Source: CAD feature listing. Evaluate the final solid. Frame: model axes, mm. A direction names the side the tool comes from. Give positions to 0.01 mm unless a question says otherwise; leave off trailing zeros. Loops run counter-clockwise (first coordinate to the right, second up) from the corner with the lowest first, then second, coordinate; pieces in that order, holes last. Notation, with made-up numbers: (-38.5, -18.5) -> (0.5, -18.5) arc R22 ccw to (0.5, -6.5) -> close; hole circle Ø7 at (72.25, 64.25). An arc over 180 degrees is marked (long way). Return JSON: item names as keys, results as strings. Group by question number.
(1) Cut plane D-D on y = -8. Return loops of the section in (x, z), then the cut area to 3 significant figures.
(2) Access query for faces 1 (the face through (0, -19, 24)), 2 (the face through (0, -21, 28)), 3 (the face through (0, 0, 54)). Directions: +Z, -Z, +X, -X, +Y, -Y. A direction counts if a zero-diameter tool reaches every point of the face in a straight line with its end or side. Return the directions, or none.
(3) Draft query along Z for faces 4 (the face through (0, -12.6, 11.5)), 5 (the face through (0, -20, 12)), 6 (the face through (0, -15, 57)). Return one class per face: released by +Z, released by -Z, zero draft, split by the parting line, or undercut.
(4) Cut plane B-B on x = 1.85. Give the number of separate pieces and of enclosed holes in the cut face, then the cut area to 3 significant figures.
(5) Cut plane A-A on y = -15. Return loops of the section in (x, z).
(6) Ray query, line 1 (Y direction, x = -1.1, z = 22.5); line 2 (Y direction, x = -0.05, z = 17); line 3 (Z direction, x = -2.1, y = -9). Return the intervals inside material, ascending. Write a range as from..to.
(7) Pin query (flat end, axial travel): pin 1 (1.5 mm diameter, centred on x = 1.5, z = 50.5, fed in from +Y); pin 2 (2 mm diameter, centred on x = 0, z = 33, fed in from +Y); pin 3 (3 mm diameter, centred on x = 1, z = 29.5, fed in from +Y). Return the tip coordinate at first contact, or that it passes through.
(8) Cut plane C-C on z = 23. Return loops of the section in (x, y), then the cut area to 3 significant figures.
Autodesk Inventor part; units mm, degrees
ref_plane "YZ Plane" through (0, 0, 0) normal (1, 0, 0) x (0, 1, 0)
ref_plane "XZ Plane" through (0, 0, 0) normal (0, 1, 0) x (-1, 0, 0)
ref_plane "XY Plane" through (0, 0, 0) normal (0, 0, 1) x (1, 0, 0)
sketch "Skizze1" plane through (0, 0, 0) normal (1, 0, 0) x (0, 1, 0)
  circle A0 centre (-22.8, 48.7) radius 11 construction
  line L0 (-97.7565, 0) -> (58.6427, 0)
  circle A1 centre (14.8, 21.5) radius 21.5 construction
  line L1 (0, 10) -> (0, 33.674) construction
  line L2 (-6.7, 0) -> (-6.7, 21.5) construction
  circle A2 centre (-4.5, 42.5) radius 5 construction
  line L3 (-56.6136, 29) -> (0, 29) construction
  line L4 (-75.4137, 30) -> (0, 30) construction
  line L5 (-21, 43.3983) -> (-29, 49)
  line L6 (-29, 49) -> (-29, 57)
  circle A3 centre (-4.5, 42.5) radius 5.5
  circle A4 centre (-22.8, 48.7) radius 0.5
  circle A5 centre (-3, 23) radius 0.8
  line L7 (14.8, 21.5) -> (-6.7, 21.5) construction
  line L8 (-29, 57) -> (0, 57)
  line L9 (14.8, 21.5) -> (14.8, 20.5) construction
  line L10 (14.8, 20.5) -> (-4.5, 42.5) construction
  circle A6 centre (-22.8, 48.7) radius 4.95 construction
  circle A7 centre (-12.2958, 49.6823) radius 5.6 construction
  circle A8 centre (-12.2958, 49.6823) radius 6.3 construction
  circle A9 centre (-12.2958, 49.6823) radius 1.525
  line L11 (0, 50.374) -> (0, 57)
  line L12 (-21, 43.3983) -> (-21, 10)
  line L13 (-21, 10) -> (0, 10)
  arc A10 (1.9876, 42.0983) -> (1.2121, 45.6019) centre (-4.5, 42.5) ccw
  line L14 (1.9876, 42.0983) -> (0, 10)
  arc A11 (0, 50.374) -> (1.2121, 45.6019) centre (10, 50.374) ccw
  line L15 (-12.5, 18) -> (-12.5, 31) construction
  line L16 (-19, 18) -> (-19, 31)
  line L17 (-6, 31) -> (-6, 18)
  arc A12 (-19, 18) -> (-6, 18) centre (-12.5, 18) ccw
  arc A13 (-6, 31) -> (-19, 31) centre (-12.5, 31) ccw
  point P0 (0, 0)
  point P1 (-12.5, 24.5)
  dimension "d4" = 43
  dimension "d0" = 22
  dimension "d6" = 6.7
  dimension "d8" = 10
  dimension "d9" = 29
  dimension "d11" = 30
  dimension "d19" = 29
  dimension "d20" = 11
  dimension "d33" = 1
  dimension "d34" = 48.7
  dimension "d36" = 1.6
  dimension "d37" = 3
  dimension "d54" = 57
  dimension "d58" = 1
  dimension "d65" = 9.9
  dimension "d66" = 11.2
  dimension "d67" = 0.7
  dimension "d68" = 3.05
  dimension "d73" = 22.8
  dimension "d100" = 10.5042
  dimension "d101" = 0.9823
  dimension "d102" = 0
  dimension "d103" = 8.3
  dimension "d104" = 21
  dimension "d107" = 10
  dimension "d110" = 8
  dimension "d111" = 55
  dimension "d112" = 13
  dimension "d113" = 10
  dimension "d114" = 42.5
  dimension "d115" = 34
  dimension "d116" = 21
  dimension "d131" = 13
  dimension "d132" = 13
  dimension "d133" = 12.5
  dimension "d134" = 18
  dimension "d135" = 4.5
  dimension "d136" = 10.55
extrude "Extrusion1" add sketch "Skizze1" along normal mid plane 5 contours L5 L6 L8 L11 A11 A10 L14 L13 L12 | A4
sketch "Skizze2" plane through (-2.5, -29, 57) normal (0, 0, 1) x (1, 0, 0)
  line L0 (0, 0) -> (5, 0)
  line L1 (5, 5) -> (5, 0)
  line L2 (0, 0) -> (0, 5)
  line L3 (2.5, 29) -> (2.5, 0) construction
  line L4 (0, 0) -> (5, 0) construction
  line L5 (0, 5) -> (5, 5)
  line L6 (0, 29) -> (5, 29)
  line L7 (0, 29) -> (5, 29)
  point P0 (2.5, 26)
  point P1 (2.5, 3)
  dimension "d25" = 23
  dimension "d74" = 3
hole "Bohrung1" at (0, -3, 57) at (0, -26, 57) direction (0, 0, -1) diameter 2.459 depth 7 tip angle 118
sketch "Skizze3" plane through (-2.5, 0, 0) normal (-1, 0, 0) x (0, 0, 1)
  circle A0 centre (23, -3) radius 0.8
  line L0 (29, -4) -> (17, -4) construction
  circle A1 centre (23, -3) radius 0.8 construction
  line L1 (23, -4) -> (23, -3) construction
  point P0 (0, 0)
  point P1 (55, -8)
  dimension "d38" = 12
  dimension "d39" = 1
  dimension "d40" = 32
  dimension "d41" = 5
hole "Bohrung2" at (-2.5, -4, 17) at (-2.5, -4, 29) at (-2.5, -8, 55) direction (1, 0, 0) diameter 1.567 end through all
fillet "Rundung3" radius 5 4 edges at (0, 0, 10) (0, -21, 10) (0, -21, 43.3983) (0, -29, 49)
properties part number "Dribbler Seite v2" material "Aluminium 6061"
Answers:
{
 "1": {"outline": "(-2.5, 10) -> (2.5, 10) -> (2.5, 13.31) -> (-2.5, 13.31) -> close; (-2.5, 35.69) -> (2.5, 35.69) -> (2.5, 38.26) -> (-2.5, 38.26) -> close; (-2.5, 46.74) -> (2.5, 46.74) -> (2.5, 54.22) -> (-2.5, 54.22) -> close; (-2.5, 55.78) -> (2.5, 55.78) -> (2.5, 57) -> (-2.5, 57) -> close", "area": "72.8 mm²"},
 "2": {"face 1": "+X, -X", "face 2": "-Z, +X, -X, -Y", "face 3": "+Z, +X, -X, +Y"},
 "3": {"face 4": "undercut", "face 5": "released by -Z", "face 6": "released by +Z"},
 "4": {"separate pieces": "1", "enclosed holes": "7", "area": "692 mm²"},
 "5": {"outline": "(-2.5, 10) -> (2.5, 10) -> (2.5, 12) -> (-2.5, 12) -> close; (-2.5, 37) -> (2.5, 37) -> (2.5, 57) -> (-2.5, 57) -> close"},
 "6": {"line 1": "-21..-19, -6..-3.62, -2.38..0.77", "line 2": "-21..-18.92, -6.08..-4.78, -3.22..0.43", "line 3": "10..12.52, 36.48..39.34, 45.66..57"},
 "7": {"pin 1": "y = 0.02", "pin 2": "y = 1.49", "pin 3": "y = 1.3"},
 "8": {"outline": "(-2.5, -21) -> (2.5, -21) -> (2.5, -19) -> (-2.5, -19) -> close; (-2.5, -6) -> (2.5, -6) -> (2.5, -3.8) -> (-2.5, -3.8) -> close; (-2.5, -2.2) -> (2.5, -2.2) -> (2.5, 0.8) -> (-2.5, 0.8) -> close", "area": "36.0 mm²"}
}
